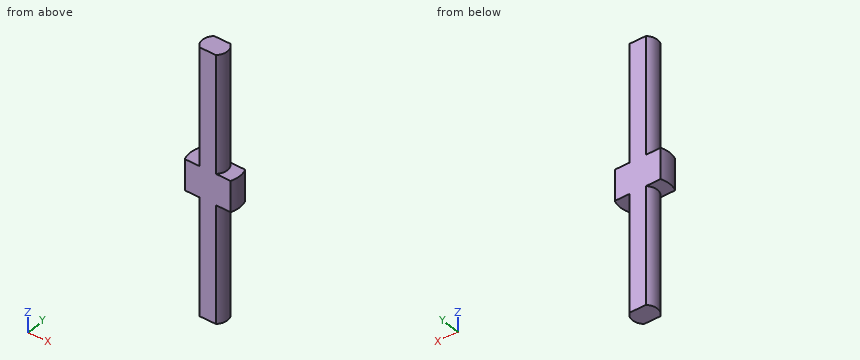
from build123d import *

# Parameters (mm, degrees)
CUT_EXTRUDE1_DEPTH      = 45.463468151
CUT_EXTRUDE1_DEPTH_BACK = 45.463468151
SKETCH2_W               = 16
SKETCH2_H               = 5


with BuildPart() as part:
    # Sketch1 → Revolve1 (revolve)
    with BuildSketch(Plane(origin=(0, 0, 0), x_dir=(1, 0, 0), z_dir=(0, 1, 0))):
        Polygon((4, 43), (4, 5), (8, 5), (8, -5), (4, -5), (4, -43), (0, -43), (0, 43), align=None)
    revolve(axis=Axis((0, 0, 43), (0, 0, -1)))

    # Sketch2 → Cut-Extrude1 (cut, two sides: drawn at the far end of the back side and taken through both)
    with BuildSketch(Plane.XY.offset(-CUT_EXTRUDE1_DEPTH_BACK)):
        with Locations((0, 5.5)):
            Rectangle(SKETCH2_W, SKETCH2_H)
        with Locations((0, -5.5)):
            Rectangle(SKETCH2_W, SKETCH2_H)
    extrude(amount=CUT_EXTRUDE1_DEPTH + CUT_EXTRUDE1_DEPTH_BACK, mode=Mode.SUBTRACT)


solid = part.part
The listing builds one solid part. Answer for the finished solid, in the listing's coordinates (mm). Round coordinates to 2 decimals unless told otherwise and drop trailing zeros. Order: outer loops, then holes, each group sorted by start corner. A loop starts at its lowest first (then second) coordinate and runs counter-clockwise, first axis right, second up. Notation, with made-up numbers: (50.5, 2) - (88.5, 2) arc R14 cw to (88.5, 28) - close; hole circle Ø6 at (-1, -16.5). An arc over 180 degrees is marked (long way). Write item = value, one per line. Start each with the question number.
1) Straight lines are drawn through the part: L1, parallel to Z at x = 5.75, y = 1.5; L2, parallel to X at y = -0.25, z = -12.5; L3, parallel to X at y = -1, z = 9.5. For each, find the intervals that lie inside material, in ascending order.
2) Section B-B, the plane z = 2.5 is taken. Write down the section's boundary in (x, y), plus the area to 3 significant figures.
3) Section A-A, the plane y = 2 is taken. Write down the section's boundary in (x, z), plus the area to 3 significant figures.
4) Given pin 1 (2 mm diameter, centred on y = -1, z = 22.5, fed in from +X); pin 2 (2.5 mm diameter, centred on x = 6.5, y = 0, fed in from +Z), each flat-ended and moving along its own axis, determine where each tip first touches the part or whether it passes through.
5) Section C-C, the plane x = -5 is taken. Write down the section's boundary in (y, z).
Results list:
q1.L1 = -5 to 5
q1.L2 = -3.99 to 3.99
q1.L3 = -3.87 to 3.87
q2.outline = (-7.42, -3) - (7.42, -3) arc R8 ccw to (7.42, 3) - (-7.42, 3) arc R8 ccw to start
q2.area = 93.7 mm^2
q3.outline = (-7.75, -5) - (-3.46, -5) - (-3.46, -43) - (3.46, -43) - (3.46, -5) - (7.75, -5) - (7.75, 5) - (3.46, 5) - (3.46, 43) - (-3.46, 43) - (-3.46, 5) - (-7.75, 5) - close
q3.area = 681 mm^2
q4.pin_1 = 4
q4.pin_2 = 5
q5.outline = (-3, -5) - (3, -5) - (3, 5) - (-3, 5) - close
